Verification items for this drawing (mm, ordinates from the low corner). Give positions to 0.01 mm unless a question says otherwise; leave off trailing zeros. Order: outer loops, then holes, each group sorted by start corner. A loop starts at its lowest first (then second) coordinate and runs counter-clockwise, first axis right, second up. Notation, with made-up numbers: M 35,-40 L 91,-40 A23 ccw 91,-11 Z; hole C 11,66 d1. An arc over 180 degrees is marked long. Answer as a JSON object with one key per item and string values.
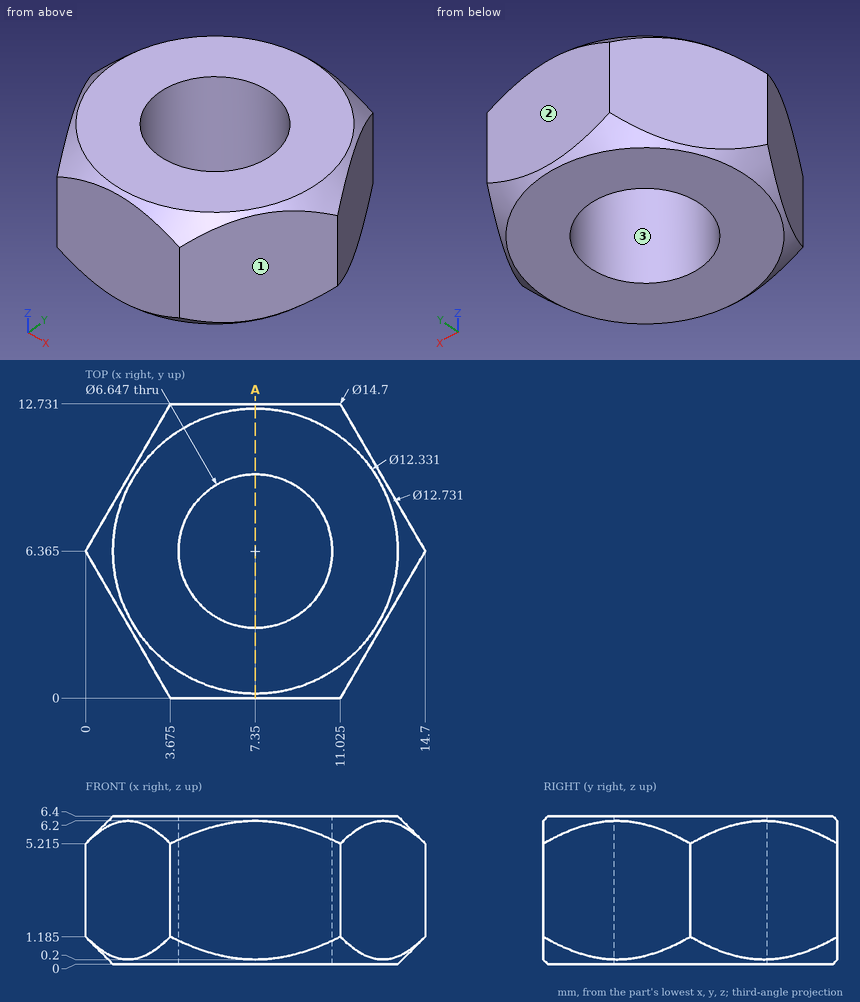
Q1. Section check A-A on x = 7.35. Record the cut outline in (y, z).
Resolved:
{"outline": "M 0,0.2 L 0.2,0 L 3.04,0 L 3.04,6.4 L 0.2,6.4 L 0,6.2 Z; M 9.69,0 L 12.53,0 L 12.73,0.2 L 12.73,6.2 L 12.53,6.4 L 9.69,6.4 Z"}
Q2. Material ranges on L1, parallel to Y at x = 10, z = 5.5; L2, parallel to Y at x = 9.75, z = 0.75 (1 decimal); L3, parallel to X at y = 8.75, z = 3.75 (1 decimal), recorded low to high.
Resolved:
{"L1": "y = 0 to 4.36, 8.37 to 12.73", "L2": "y = 0 to 4.1, 8.7 to 12.7", "L3": "x = 1.4 to 5, 9.7 to 13.3"}
Q3. Release check for a two-part mould opening along X. For the marked faces 1, 2 and 3 record: +X half, -X half, draft (parallel to the pull), parting line (faces both ways), or undercut.
Resolved:
{"face 1": "+X half", "face 2": "draft", "face 3": "undercut"}
Q4. Gauge pin test, flat end, axial feed: pin 1 Ø4 at (x, y) = (8, 3.5) entering from +Z. Record the tip position at first contact, or that the pin passes through.
Resolved:
{"pin 1": "stops at z = 6.4"}
